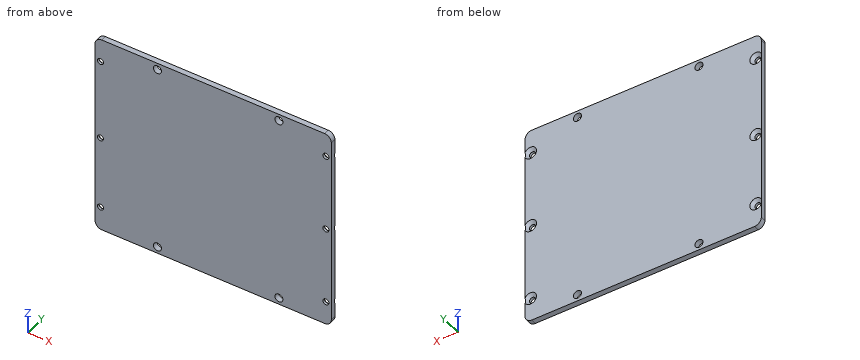
```python
from build123d import *

# Parameters (mm, degrees)
IZIM1_W                       = 175
IZIM1_H                       = 150
Y_KSEKLIK_EKSTR_ZYON1_DEPTH   = 4
RADYUS1_R                     = 5
IZIM2_R                       = 2
IZIM2_R_2                     = 3
KES_EKSTR_ZYON1_DEPTH         = 10
M4_SFHCS_IN_HAV_A1_AT_2_COUNT = 2
M4_SFHCS_IN_HAV_A1_AT_2_PITCH = 54.690877802
M4_SFHCS_IN_HAV_A1_AT_3_COUNT = 2
M4_SFHCS_IN_HAV_A1_AT_3_PITCH = 115
M4_SFHCS_IN_HAV_A1_AT_4_COUNT = 2
M4_SFHCS_IN_HAV_A1_AT_4_PITCH = 202.765874841
M4_SFHCS_IN_HAV_A1_AT_5_COUNT = 2
M4_SFHCS_IN_HAV_A1_AT_5_PITCH = 176.621771025
M4_SFHCS_IN_HAV_A1_AT_6_COUNT = 2
M4_SFHCS_IN_HAV_A1_AT_6_PITCH = 167


with BuildPart() as part:
    # Çizim1 → Yükseklik-Ekstrüzyon1 (new body)
    with BuildSketch(Plane(origin=(0, 0, 0), x_dir=(1, 0, 0), z_dir=(0, 1, 0))):
        Rectangle(IZIM1_W, IZIM1_H)
    extrude(amount=Y_KSEKLIK_EKSTR_ZYON1_DEPTH)

    # Radyus1
    radyus1_edges = [part.edges().sort_by_distance(p)[0] for p in [
        (-87.5, 2, -75),
        (87.5, 2, -75),
        (87.5, 2, 75),
        (-87.5, 2, 75),
    ]]
    fillet(radyus1_edges, radius=RADYUS1_R)

    # Çizim2 → Kes-Ekstrüzyon1 (cut)
    with BuildSketch(Plane(origin=(0, 4, 0), x_dir=(1, 0, 0), z_dir=(0, 1, 0))):
        with Locations(Location((-83.5, -57.5, 0), (0, 0, 270))):
            Circle(IZIM2_R)
        with Locations(Location((83.5, -57.5, 0), (0, 0, 270))):
            Circle(IZIM2_R)
        with Locations(Location((83.5, 0, 0), (0, 0, 270))):
            Circle(IZIM2_R)
        with Locations(Location((83.5, 57.5, 0), (0, 0, 270))):
            Circle(IZIM2_R)
        with Locations(Location((-83.5, 57.5, 0), (0, 0, 270))):
            Circle(IZIM2_R)
        with Locations(Location((-83.5, 2.809122198, 0), (0, 0, 270))):
            Circle(IZIM2_R)
        with Locations(Location((-41.307504104, -70, 0), (0, 0, 270))):
            Circle(IZIM2_R_2)
        with Locations(Location((48.692495896, -70, 0), (0, 0, 270))):
            Circle(IZIM2_R_2)
        with Locations(Location((-41.307504104, 70, 0), (0, 0, 270))):
            Circle(IZIM2_R_2)
        with Locations(Location((48.692495896, 70, 0), (0, 0, 270))):
            Circle(IZIM2_R_2)
    extrude(amount=-KES_EKSTR_ZYON1_DEPTH, mode=Mode.SUBTRACT)

    # Çizim3 → M4 SFHCS İçin Havşa1 (revolve, cut)
    with BuildSketch(Plane(origin=(-83.5, 4, -57.5), x_dir=(0, 0, 1), z_dir=(1, 0, 0))):
        Polygon((0, 0), (0, 4), (2.25, 4), (2.25, 2.23), (4.48, 0), align=None)
    m4_sfhcs_in_hav_a1 = revolve(axis=Axis((-83.5, 10.35, -57.5), (0, -1, 0)), mode=Mode.SUBTRACT)

    # M4 SFHCS İçin Havşa1 at 2: M4 SFHCS İçin Havşa1 ×2
    with Locations(*[(0, 0, i * M4_SFHCS_IN_HAV_A1_AT_2_PITCH) for i in range(1, M4_SFHCS_IN_HAV_A1_AT_2_COUNT)]):
        add(m4_sfhcs_in_hav_a1, mode=Mode.SUBTRACT)

    # M4 SFHCS İçin Havşa1 at 3: M4 SFHCS İçin Havşa1 ×2
    with Locations(*[(0, 0, i * M4_SFHCS_IN_HAV_A1_AT_3_PITCH) for i in range(1, M4_SFHCS_IN_HAV_A1_AT_3_COUNT)]):
        add(m4_sfhcs_in_hav_a1, mode=Mode.SUBTRACT)

    # M4 SFHCS İçin Havşa1 at 4: M4 SFHCS İçin Havşa1 ×2
    with Locations(*[Vector(0.8236099892599149, 0, 0.5671565794304804) * (i * M4_SFHCS_IN_HAV_A1_AT_4_PITCH) for i in range(1, M4_SFHCS_IN_HAV_A1_AT_4_COUNT)]):
        add(m4_sfhcs_in_hav_a1, mode=Mode.SUBTRACT)

    # M4 SFHCS İçin Havşa1 at 5: M4 SFHCS İçin Havşa1 ×2
    with Locations(*[Vector(0.9455233011811556, 0, 0.3255544300474038) * (i * M4_SFHCS_IN_HAV_A1_AT_5_PITCH) for i in range(1, M4_SFHCS_IN_HAV_A1_AT_5_COUNT)]):
        add(m4_sfhcs_in_hav_a1, mode=Mode.SUBTRACT)

    # M4 SFHCS İçin Havşa1 at 6: M4 SFHCS İçin Havşa1 ×2
    with Locations(*[(i * M4_SFHCS_IN_HAV_A1_AT_6_PITCH, 0, 0) for i in range(1, M4_SFHCS_IN_HAV_A1_AT_6_COUNT)]):
        add(m4_sfhcs_in_hav_a1, mode=Mode.SUBTRACT)


solid = part.part
```
Model file for the job. Use its own axes, mm. Round coordinates to 2 decimals unless told otherwise and drop trailing zeros. Write each loop counter-clockwise with the first axis right and the second up, starting at its lowest first coordinate (ties: lowest second). Pieces come first, ordered by that corner, then holes. Notation, with made-up numbers: M 13.25,69 L 61.25,69 A25 cw 61.25,93 Z; hole C 85.5,54.5 d10. An arc over 180 degrees is marked long. Put each result on its own line as item: value.
Item 1: Cut at B-B (y = 3.25). State how many separate pieces and enclosed holes the cut face has, and give its area (3 significant figures).
Responses:
separate pieces: 1
enclosed holes: 10
area: 25,900 mm²
Item 2: Flat gauge pin, fed straight in: P1, Ø6, axis at x = 83.5, z = 57.5, coming from the +Y side. Where does the tip first touch, or does it go through?
Responses:
P1: y = 2.52
Item 3: Cut at A-A (z = 57.5). List the corners of the cut face in (x, y), and give its area (3 significant figures).
Responses:
outline: M -87.5,0 L -85.75,0 L -85.75,1.77 L -87.5,3.52 Z; M -81.25,0 L 81.25,0 L 81.25,1.77 L 79.02,4 L -79.02,4 L -81.25,1.77 Z; M 85.75,0 L 87.5,0 L 87.5,3.52 L 85.75,1.77 Z
area: 654 mm²
Item 4: Probe L1, parallel to X at y = 0.85, z = 57.5; L2, parallel to Z at x = -83.5, y = 1.1; L3, parallel to X at y = 0.95, z = 70. List the from-to ranges inside material, lowest first. Write a range as from..to.
Responses:
L1: -87.5..-85.75, -81.25..81.25, 85.75..87.5
L2: -74.9..-59.75, -55.25..-5.06, -0.56..55.25, 59.75..74.9
L3: -87.5..-44.31, -38.31..45.69, 51.69..87.5
